Source: CAD feature listing. Evaluate the final solid. Frame: model axes, mm. Face numbers are marked on the shaded views. A direction names the side the tool comes from. Give positions to 0.01 mm unless a question says otherwise; leave off trailing zeros. Write each loop counter-clockwise with the first axis right and the second up, starting at its lowest first coordinate (ties: lowest second). Pieces come first, ordered by that corner, then holes. Notation, with made-up numbers: (24.5, 40.25) -> (79.5, 40.25) arc R33 cw to (79.5, 68.25) -> close; hole circle Ø5 at (76, 48). An arc over 180 degrees is marked (long way). Write item = value, one per line.
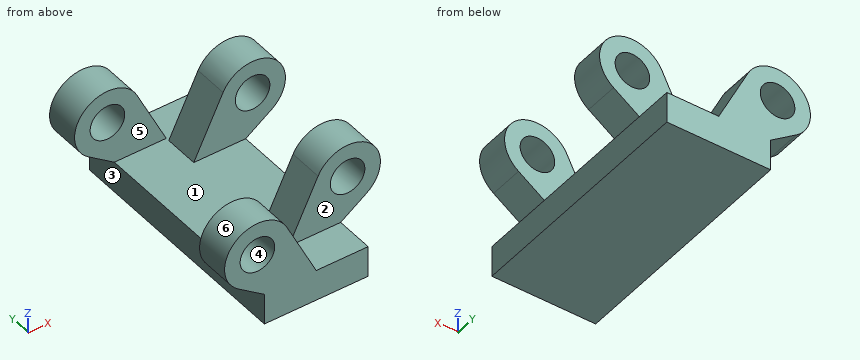
from build123d import *

# Parameters (mm, degrees)
EXTRUDE_1_DEPTH          = 7
EXTRUDE_1_DEPTH_BACK     = 7
SKETCH_1_W               = 6
SKETCH_1_H               = 1.8
SKETCH_1_R               = 1.9
SKETCH_1_R_2             = 1
CUT_EXTRUDE_1_DEPTH      = 5
CUT_EXTRUDE_1_DEPTH_BACK = 5
CUT_EXTRUDE_2_DEPTH      = 2.8
CUT_EXTRUDE_2_DEPTH_BACK = 2.8
CUT_EXTRUDE_START        = -2.2
CUT_EXTRUDE_3_DEPTH      = 2.2


with BuildPart() as part:
    # Sketch 1 → Extrude 1 (new, two sides: drawn at the far end of the back side and taken through both)
    # profile 1 of 5: a face of its own
    with BuildSketch(Plane(origin=(0, 0, 0), x_dir=(1, 0, 0), z_dir=(0, 1, 0)).offset(-EXTRUDE_1_DEPTH_BACK)):
        with Locations((3, -0.9)):
            Rectangle(SKETCH_1_W, SKETCH_1_H)
    # profile 2 of 5: a face of its own
    with BuildSketch(Plane(origin=(0, 0, 0), x_dir=(1, 0, 0), z_dir=(0, 1, 0)).offset(-EXTRUDE_1_DEPTH_BACK)):
        with BuildLine():
            Line((3, -1.8), (0, -1.8))
            Line((0, -1.8), (-1.490107264, -2.843829652))
            ThreePointArc((-1.490107264, -2.843829652), (0.477153407, -2.714591474), (1.5, -4.4))
            ThreePointArc((1.5, -4.4), (1.450399061, -4.831304204), (1.304185983, -5.240089362))
            Line((1.304185983, -5.240089362), (3, -1.8))
        make_face()
    # profile 3 of 5: a face of its own
    with BuildSketch(Plane(origin=(0, 0, 0), x_dir=(1, 0, 0), z_dir=(0, 1, 0)).offset(-EXTRUDE_1_DEPTH_BACK)):
        with BuildLine():
            Line((6, -1.8), (3, -1.8))
            Line((3, -1.8), (4.695814017, -5.240089362))
            ThreePointArc((4.695814017, -5.240089362), (5.163153883, -2.957706104), (7.490107264, -2.843829652))
            Line((7.490107264, -2.843829652), (6, -1.8))
        make_face()
    # profile 4 of 5: a face of its own
    with BuildSketch(Plane(origin=(0, 0, 0), x_dir=(1, 0, 0), z_dir=(0, 1, 0)).offset(-EXTRUDE_1_DEPTH_BACK)):
        with Locations((6.4, -4.4)):
            Circle(SKETCH_1_R)
        with Locations(Location((6.4, -4.4, 0), (0, 0, 270))):
            Circle(SKETCH_1_R_2, mode=Mode.SUBTRACT)
    # profile 5 of 5: a face of its own
    with BuildSketch(Plane(origin=(0, 0, 0), x_dir=(1, 0, 0), z_dir=(0, 1, 0)).offset(-EXTRUDE_1_DEPTH_BACK)):
        with Locations((-0.4, -4.4)):
            Circle(SKETCH_1_R)
        with Locations(Location((-0.4, -4.4, 0), (0, 0, 270))):
            Circle(SKETCH_1_R_2, mode=Mode.SUBTRACT)
    extrude(amount=EXTRUDE_1_DEPTH + EXTRUDE_1_DEPTH_BACK)

    # Sketch 2 → Cut-Extrude 1 (cut, two sides: drawn at the far end of the back side and taken through both)
    with BuildSketch(Plane(origin=(0, 0, 0), x_dir=(1, 0, 0), z_dir=(0, 1, 0)).offset(-CUT_EXTRUDE_1_DEPTH_BACK)):
        with BuildLine():
            Line((0, -1.8), (3, -1.8))
            Line((3, -1.8), (1.304185983, -5.240089362))
            ThreePointArc((1.304185983, -5.240089362), (-1.636846117, -5.842293896), (-1.490107264, -2.843829652))
            Line((-1.490107264, -2.843829652), (0, -1.8))
        make_face()
    extrude(amount=CUT_EXTRUDE_1_DEPTH + CUT_EXTRUDE_1_DEPTH_BACK, mode=Mode.SUBTRACT)

    # Sketch 3 → Cut-Extrude 2 (cut, two sides: drawn at the far end of the back side and taken through both)
    with BuildSketch(Plane(origin=(0, 0, 0), x_dir=(1, 0, 0), z_dir=(0, 1, 0)).offset(-CUT_EXTRUDE_2_DEPTH_BACK)):
        with BuildLine():
            Line((4.695814017, -5.240089362), (3, -1.8))
            Line((3, -1.8), (6, -1.8))
            Line((6, -1.8), (7.490107264, -2.843829652))
            ThreePointArc((7.490107264, -2.843829652), (7.636846117, -5.842293896), (4.695814017, -5.240089362))
        make_face()
    extrude(amount=CUT_EXTRUDE_2_DEPTH + CUT_EXTRUDE_2_DEPTH_BACK, mode=Mode.SUBTRACT)

    # Sketch 4 → Cut-Extrude 3 (cut)
    with BuildSketch(Plane(origin=(0, 7, 0), x_dir=(1, 0, 0), z_dir=(0, 1, 0)).offset(CUT_EXTRUDE_START)):
        with BuildLine():
            Line((7.490107264, -2.843829652), (6, -1.8))
            Line((6, -1.8), (3, -1.8))
            Line((3, -1.8), (4.695814017, -5.240089362))
            ThreePointArc((4.695814017, -5.240089362), (7.636846117, -5.842293896), (7.490107264, -2.843829652))
        make_face()
    cut_extrude_3 = extrude(amount=CUT_EXTRUDE_3_DEPTH, mode=Mode.SUBTRACT)

    # Mirror 1: Cut-Extrude 3 across plane
    add(cut_extrude_3.mirror(Plane.ZX), mode=Mode.SUBTRACT)


solid = part.part
1) Draft query along Z for the marked faces 4, 5 and 6. Return one class per face: pulls with the +Z half, pulls with the -Z half, needs draft (parallel to the pull), parting line crosses it, or undercut.
Computed:
face_4 = undercut
face_5 = needs draft
face_6 = parting line crosses it
2) Cut plane C-C (x = -1). Return the cut outline in (y, z), then the cut area to 3 significant figures.
Computed:
outline = (-7, 2.5) -> (-5, 2.5) -> (-5, 3.6) -> (-7, 3.6) -> close; (-7, 5.2) -> (-5, 5.2) -> (-5, 6.2) -> (-7, 6.2) -> close; (5, 2.5) -> (7, 2.5) -> (7, 3.6) -> (5, 3.6) -> close; (5, 5.2) -> (7, 5.2) -> (7, 6.2) -> (5, 6.2) -> close
area = 8.41 mm²
3) Cut plane A-A (y = -5.75). Return the cut outline in (x, z).
Computed:
outline = (-1.49, 2.84) -> (0, 1.8) -> (0, 0) -> (6, 0) -> (6, 1.8) -> (3, 1.8) -> (1.3, 5.24) arc R1.9 ccw (long way) to start; hole circle Ø2 at (-0.4, 4.4)
4) Access query for the marked faces 1, 2 and 3. Directions: +Z, -Z, +X, -X, +Y, -Y. A direction counts if a zero-diameter tool reaches every point of the face in a straight line with its end or side. Return the directions, or none.
Computed:
face_1 = +Z
face_2 = +Z, +X, -X, -Y
face_3 = -Z, -X, +Y, -Y
5) Cut plane D-D (x = 0.25). Return the cut outline in (y, z), then the cut area to 3 significant figures.
Computed:
outline = (-7, 0) -> (7, 0) -> (7, 3.64) -> (5, 3.64) -> (5, 1.8) -> (-5, 1.8) -> (-5, 3.64) -> (-7, 3.64) -> close; (-7, 5.16) -> (-5, 5.16) -> (-5, 6.19) -> (-7, 6.19) -> close; (5, 5.16) -> (7, 5.16) -> (7, 6.19) -> (5, 6.19) -> close
area = 36.7 mm²
6) Contact query for flat-ended pins moving along their axis: pin 1 (1.6 mm diameter, centred on x = 6.4, z = 4.4, fed in from -Y); pin 2 (2 mm diameter, centred on y = 2, z = 1.5, fed in from -X); pin 3 (1.5 mm diameter, centred on y = 3, z = 5, fed in from -X); pin 4 (1.4 mm diameter, centred on y = 1, z = 1, fed in from +X). Output: stop coordinate, or through.
Computed:
pin_1 = through
pin_2 = 0
pin_3 = 4.21
pin_4 = 6
7) Cut plane B-B (z = 4.5). State how many separate pieces and enclosed holes the cut face has, then the cut area to 3 significant figures.
Computed:
separate_pieces = 8
enclosed_holes = 0
area = 15.8 mm²
8) Material intervals for L1, parallel to Y at x = 5, z = 2; L2, parallel to Y at x = 0, z = 3.25; L3, parallel to Z at x = 6.4, y = 3.45, sorted ascending.
Computed:
L1 = -4.8 to -2.8, 2.8 to 4.8
L2 = -7 to -5, 5 to 7
L3 = 2.08 to 3.4, 5.4 to 6.3
